```python
from build123d import *

# Parameters (mm, degrees)
F0_W     = 57.15
F0_H     = 44.45
F1_DEPTH = 25.4
F3_DEPTH = 25.401
F5_DEPTH = 12.7


with BuildPart() as f1:
    # F0 (on Front) → F1 (new body)
    with BuildSketch(Plane.XZ):
        with Locations((1.4072097838, 9.1718252664)):
            Rectangle(F0_W, F0_H)
    extrude(amount=F1_DEPTH)

    # F2 (on face) → F3 (cut, through all)
    with BuildSketch(Plane.XZ.offset(25.4)):
        with BuildLine():
            ThreePointArc((-1.7677901676, 25.0468252664), (-10.7480463069, 21.3270814178), (-14.4677902162, 12.3468253036))
            ThreePointArc((-14.4677902162, 12.3468253036), (-10.7480463548, 3.3665691629), (-1.7677902287, -0.3531747336))
            ThreePointArc((-1.7677902287, -0.3531747336), (7.2124659004, 3.3665691409), (10.9322097838, 12.3468252664))
            ThreePointArc((10.9322097838, 12.3468252664), (7.2124659221, 21.3270813703), (-1.7677901676, 25.0468252664))
        make_face()
    extrude(amount=-F3_DEPTH, mode=Mode.SUBTRACT)

    # F4 (on face) → F5 (cut)
    with BuildSketch(Plane.XZ.offset(25.4)):
        with BuildLine():
            Line((29.9822097838, 31.3968252664), (-8.1177902162, 31.3968252664))
            Line((-8.1177902162, 31.3968252664), (-4.3389383209, 24.7838344496))
            ThreePointArc((-4.3389383209, 24.7838344496), (6.25207322, 22.1942508419), (10.9322097838, 12.3468252664))
            ThreePointArc((10.9322097838, 12.3468252664), (10.0810924836, 7.7758320739), (7.641819427, 3.8175083909))
            Line((7.641819427, 3.8175083909), (17.2822097838, -13.0531747336))
            Line((17.2822097838, -13.0531747336), (29.9822097838, -13.0531747336))
            Line((29.9822097838, -13.0531747336), (29.9822097838, 31.3968252664))
        make_face()
    extrude(amount=-F5_DEPTH, mode=Mode.SUBTRACT)


solid = f1.part
```
Geometry: final body of the model. Coordinates: model frame, mm. A direction names the side the tool comes from. Round coordinates to 2 decimals unless told otherwise and drop trailing zeros. Loops run counter-clockwise (first coordinate to the right, second up) from the corner with the lowest first, then second, coordinate; pieces in that order, holes last. Notation, with made-up numbers: (19, 33.25) -> (46, 33.25) arc R6 ccw to (46, 44.25) -> close; hole circle Ø7 at (-7.75, 85). An arc over 180 degrees is marked (long way). Use one line per item in the form item = value. Start each with the question number.
1) Section A-A on y = -2. Output: boundary loops of the cut face in (x, z), then the cut area to 3 significant figures.
2) Section C-C on x = 9. Output: boundary loops of the cut face in (y, z), then the cut area to 3 significant figures.
3) Line query: L1, parallel to X at y = -9.25, z = 12; L2, parallel to X at y = -2.5, z = 16.5; L3, parallel to Y at x = 23.5, z = 12.5. Output: solid intervals per line, ascending.
4) Access query for faces 1 (the flat face through (-27.168, -13, 9)), 2 (the flat face through (-6.255, -19.139, 28.137)). Directions: +Z, -Z, +X, -X, +Y, -Y. A direction counts if a zero-diameter tool reaches every point of the face in a straight line with its end or side. Return the directions, or none.
5) Section B-B on z = 22.5. Output: boundary loops of the cut face in (x, y).
6) Section D-D on y = -14.75. Output: boundary loops of the cut face in (x, z).
7) First-contact query: P1, Ø2, axis at x = 24, z = -8, coming from the -Y side. Flat tip, straight axial feed; report the tip coordinate or a pass-through.
Response:
q1.outline = (-27.17, -13.05) -> (29.98, -13.05) -> (29.98, 31.4) -> (-27.17, 31.4) -> close; hole circle Ø25.4 at (-1.77, 12.35)
q1.area = 2,030 mm^2
q2.outline = (-25.4, -13.05) -> (0, -13.05) -> (0, 5.61) -> (-12.7, 5.61) -> (-12.7, 1.44) -> (-25.4, 1.44) -> close; (-12.7, 19.08) -> (0, 19.08) -> (0, 31.4) -> (-12.7, 31.4) -> close
q2.area = 578 mm^2
q3.L1 = -27.17 to -14.46, 10.93 to 29.98
q3.L2 = -27.17 to -13.77, 10.23 to 29.98
q3.L3 = -12.7 to 0
q4.face_1 = +Z, -Z, -X, +Y, -Y
q4.face_2 = +Z, +X, -Y
q5.outline = (-27.17, -25.4) -> (-9.4, -25.4) -> (-9.4, 0) -> (-27.17, 0) -> close; (5.86, -12.7) -> (29.98, -12.7) -> (29.98, 0) -> (5.86, 0) -> close
q6.outline = (-27.17, -13.05) -> (17.28, -13.05) -> (7.64, 3.82) arc R12.7 cw (long way) to (-4.34, 24.78) -> (-8.12, 31.4) -> (-27.17, 31.4) -> close
q7.P1 = -12.7
